The model under review builds one solid part; all positions refer to its coordinate system, in mm. A direction names the side the tool comes from. Round coordinates to 2 decimals unless told otherwise and drop trailing zeros. Write each loop counter-clockwise with the first axis right and the second up, starting at its lowest first coordinate (ties: lowest second). Pieces come first, ordered by that corner, then holes. Notation, with made-up numbers: (29.25, -36) -> (58.25, -36) arc R24 cw to (58.25, -10) -> close; hole circle Ø3 at (15.25, 21.25). An arc over 180 degrees is marked (long way). Answer as a JSON object with one key per item and string values. Group by question number.
1) To check wall thickness, follow probe 1 along Z at (x, y) = (0, 2); probe 2 along Z at (x, y) = (-82.5, 2.5); probe 3 along X at (y, z) = (24.5, 2). State the ranges of each line that lie inside material, in increasing order. Write a range as [from, to].
2) Mouldability with a two-part tool opening along Z and no side actions: class faces 4 (the cylindrical face through (130.34, 26.06, -41.05)), 5 (the cylindrical face through (110.86, 22.54, 85.01)), 6 (the cylindrical face through (108.113, 0.711, -34.047)), 7 (the flat face through (25, -2.032, -111)) as pulls with the +Z half, pulls with the -Z half, needs draft (parallel to the pull), parting line crosses it, or undercut.
3) We need section C-C, the plane x = -63.5. Write out the cut boundary in (y, z), then the cut area to 3 significant figures.
4) Machinability: for faces 1 (the flat face through (-134, 45.72, -30)), 2 (the flat face through (28, 5.842, -2)), 3 (the flat face through (-2, 3.378, -24)), which of the approach directions +Z, -Z, +X, -X, +Y, -Y give a long, thin tool a straight path to every point of the face, cutting with its end or side? Answer none if there is none.
5) We need section D-D, the plane y = 17. Write out the cut boundary in (x, z).
6) Insertion check: pin 1 Ø3 at (x, z) = (-5.5, 66.5) entering from +Y; pin 2 Ø10 at (x, y) = (-11, 35.5) entering from +Z; pin 3 Ø2 at (y, z) = (11.5, 67.5) entering from -X. Each pin has a flat end and moves straight along its axis. Give the tip position at first contact, or say it passes through.
7) We need section A-A, the plane x = 0. Write out the cut boundary in (y, z), then the cut area to 3 significant figures.
8) We need section B-B, the plane z = 0. Count the separate pieces of the cut face and the enclosed holes in it, then the cut area to 3 significant figures.
Autodesk Inventor part; units mm, degrees
ref_plane "YZ Plane" through (0, 0, 0) normal (1, 0, 0) x (0, 1, 0)
ref_plane "XZ Plane" through (0, 0, 0) normal (0, 1, 0) x (-1, 0, 0)
ref_plane "XY Plane" through (0, 0, 0) normal (0, 0, 1) x (1, 0, 0)
sketch "Sketch1" plane through (0, 0, 0) normal (0, 1, 0) x (-1, 0, 0)
  circle A0 centre (0, 0) radius 139.7
  dimension "d0" = 279.4
extrude "Extrusion1" add sketch "Sketch1" along normal blind 45.72
sketch "Sketch3" plane through (0, 45.72, 0) normal (0, 1, 0) x (1, 0, 0)
  circle A0 centre (0, 0) radius 136.652
  dimension "d7" = 273.304
extrude "Extrusion3" cut sketch "Sketch3" against normal blind 39.878
sketch "Sketch4" plane through (0, 0, 0) normal (0, -1, 0) x (1, 0, 0)
  circle A0 centre (0, 0) radius 137.16
  dimension "d10" = 274.32
extrude "Extrusion5" cut sketch "Sketch4" against normal blind 3.3782
sketch "Sketch5" plane through (0, 3.3782, 0) normal (0, -1, 0) x (1, 0, 0)
  circle A0 centre (0, 0) radius 115.8875
  circle A1 centre (0, 0) radius 113.3475
  dimension "d15" = 231.775
  dimension "d16" = 226.695
extrude "Extrusion6" add sketch "Sketch5" along normal blind 5.4102
sketch "Sketch6" plane through (0, 5.842, 0) normal (0, 1, 0) x (1, 0, 0)
  circle A0 centre (0, 0) radius 6.35
  dimension "d19" = 12.7
extrude "Extrusion7" cut sketch "Sketch6" against normal through all
sketch "Sketch7" plane through (0, 5.842, 0) normal (0, -1, 0) x (1, 0, 0)
  point P0 (0, 0)
  point P1 (127, 0)
  point P2 (63.5, 109.9852)
  point P3 (-63.5, 109.9852)
  point P4 (-127, 0)
  point P5 (-63.5, -109.9852)
  point P6 (63.5, -109.9852)
  dimension "d22" = 127
  dimension "d25" = 360
hole "Hole1" at (127, 5.842, 0) at (63.5, 5.842, 109.9852) at (-63.5, 5.842, 109.9852) at (-127, 5.842, 0) at (-63.5, 5.842, -109.9852) at (63.5, 5.842, -109.9852) direction (0, -1, 0) diameter 6.604 end through all countersink diameter 12.5984 countersink angle 90
sketch "Sketch8" plane through (0, 3.3782, 0) normal (0, -1, 0) x (1, 0, 0)
  point P0 (0, 0)
properties part number "bowl"
Here are the results:
{
 "1": {"probe 1": "z = [-139.7, -137.16], [-115.89, -113.35], [113.35, 115.89], [137.16, 139.7]", "probe 2": "z = [-112.74, -109.57], [-81.39, -77.73], [77.73, 81.39], [109.57, 112.74]", "probe 3": "x = [-139.69, -136.64], [136.64, 139.69]"},
 "2": {"face 4": "undercut", "face 5": "parting line crosses it", "face 6": "undercut", "face 7": "needs draft"},
 "3": {"outline": "(-2.03, -96.94) -> (3.38, -96.94) -> (3.38, -106.15) -> (5.84, -103.69) -> (5.84, 103.69) -> (3.38, 106.15) -> (3.38, 96.94) -> (-2.03, 96.94) -> (-2.03, 93.89) -> (3.38, 93.89) -> (3.38, -93.89) -> (-2.03, -93.89) -> close; (0, -124.43) -> (45.72, -124.43) -> (45.72, -121) -> (5.84, -121) -> (5.84, -116.28) -> (3.38, -113.82) -> (3.38, -121.58) -> (0, -121.58) -> close; (0, 121.58) -> (3.38, 121.58) -> (3.38, 113.82) -> (5.84, 116.28) -> (5.84, 121) -> (45.72, 121) -> (45.72, 124.43) -> (0, 124.43) -> close", "area": "889 mm^2"},
 "4": {"face 1": "+Z, -Z, +X, -X, +Y", "face 2": "+Y", "face 3": "-Y"},
 "5": {"outline": "circle Ø279.4 at (0, 0); hole circle Ø273.3 at (0, 0)"},
 "6": {"pin 1": "stops at y = 5.84", "pin 2": "stops at z = 139.57", "pin 3": "stops at x = -122.86"},
 "7": {"outline": "(-2.03, -115.89) -> (3.38, -115.89) -> (3.38, -137.16) -> (0, -137.16) -> (0, -139.7) -> (45.72, -139.7) -> (45.72, -136.65) -> (5.84, -136.65) -> (5.84, -6.35) -> (3.38, -6.35) -> (3.38, -113.35) -> (-2.03, -113.35) -> close; (-2.03, 113.35) -> (3.38, 113.35) -> (3.38, 6.35) -> (5.84, 6.35) -> (5.84, 136.65) -> (45.72, 136.65) -> (45.72, 139.7) -> (0, 139.7) -> (0, 137.16) -> (3.38, 137.16) -> (3.38, 115.89) -> (-2.03, 115.89) -> close", "area": "945 mm^2"},
 "8": {"separate pieces": "4", "enclosed holes": "0", "area": "895 mm^2"}
}
